Geometry: final body of the model. Coordinates: model frame, mm. Face numbers are marked on the shaded views. Coordinates: 2 decimals unless noted, no trailing zeros. Write each loop counter-clockwise with the first axis right and the second up, starting at its lowest first coordinate (ties: lowest second). Pieces come first, ordered by that corner, then holes. Notation, with made-up numbers: (-27.75, 82) -> (16.25, 82) arc R18 cw to (16.25, 89) -> close; hole circle Ø11 at (80, -23). An arc over 180 degrees is marked (long way). One line per item, written item: value.
```python
from build123d import *

# Parameters (mm, degrees)
F0_W      = 76.2
F0_H      = 146.05
F1_DEPTH  = 12.7
F2_R      = 5.08
F3_R      = 5.08
F4_DEPTH  = 2.54
F5_W      = 2.4973305091
F5_H      = 11.7452070117
F5_W_2    = 2.54
F5_W_3    = 2.9405460703
F6_DEPTH  = 2.54
F7_W      = 2.8808997013
F7_H      = 5.0969719887
F8_DEPTH  = 2.032
F9_W      = 1.4404498506
F9_H      = 5.0969719887
F10_DEPTH = 3.048
F11_W     = 2.54
F11_H     = 11.43
F12_DEPTH = 1.016
F13_W     = 2.54
F13_H     = 11.43
F14_DEPTH = 1.016
F16_DEPTH = 0.508
F17_W     = 15.7348513603
F17_H     = 10.4662538506
F17_H_2   = 4.2268524888
F18_DEPTH = 2.286
F19_W     = 18.1282758713
F19_H     = 1.7902922965
F19_H_2   = 2.54
F19_H_3   = 2.6172961119
F20_DEPTH = 2.286
F21_R     = 2.1027824112
F22_DEPTH = 2.286
F24_DEPTH = 1.27
F25_W     = 13.5468328476
F25_H     = 1.6100406647
F4_FACE_W = 66.04
F4_FACE_H = 135.89
F4_FACE_R = 6.0325
F26_DEPTH = 0.508
F27_R     = 1.3953400064
F28_DEPTH = 0.508
F30_DEPTH = 0.508
F31_W     = 6.604
F31_H     = 3.0624943002
F31_H_2   = 5.8275056998
F31_H_3   = 2.54
F32_DEPTH = 2.286
F34_DEPTH = 1.27
F35_W     = 24.4420864832
F35_H     = 11.2134301376
F36_DEPTH = 2.286
F39_R     = 2.3136513578
F40_DEPTH = 0.254
F42_DEPTH = 1.016
F43_DEPTH = 1.778
F44_W     = 2.54
F44_H     = 8.934661746
F45_DEPTH = 1.016


# Not quite as in the source:
# - the program builds the solid bodies; features that only make, move or delete a surface that nothing else refers to are left out


with BuildPart() as f1:
    # F0 (on Front) → F1 (new body)
    with BuildSketch(Plane.XZ):
        with Locations((38.1, 73.025)):
            Rectangle(F0_W, F0_H)
    extrude(amount=F1_DEPTH)

    # F2
    f2_edges = [f1.edges().sort_by_distance(p)[0] for p in [
        (0, -12.7, 73.025),
        (38.1, -12.7, 0),
        (76.2, -12.7, 73.025),
        (38.1, -12.7, 146.05),
    ]]
    fillet(f2_edges, radius=F2_R)

    # F3
    f3_edges = [f1.edges().sort_by_distance(p)[0] for p in [
        (0, 0, 73.025),
        (38.1, 0, 0),
        (76.2, 0, 73.025),
        (38.1, 0, 146.05),
    ]]
    fillet(f3_edges, radius=F3_R)

    # F4 (cut): a face of the model
    f4_faces = [f1.faces().sort_by_distance(p)[0] for p in [
        (38.1, -12.7, 73.025),
    ]]
    extrude(f4_faces, amount=-F4_DEPTH, mode=Mode.SUBTRACT)

    # F5 (on face) → F6 (cut)
    with BuildSketch(Plane(origin=(0, 0, 0), x_dir=(0, -1, 0), z_dir=(-1, 0, 0))):
        with Locations((3.8313347455, 127.8729029)):
            Rectangle(F5_W, F5_H)
        with Locations((6.35, 127.8729029)):
            Rectangle(F5_W_2, F5_H)
        with Locations((9.0902730352, 127.8729029)):
            Rectangle(F5_W_3, F5_H)
    extrude(amount=-F6_DEPTH, mode=Mode.SUBTRACT)

    # F7 (on face) → F8 (join)
    with BuildSketch(Plane(origin=(2.54, 0, 0), x_dir=(0, -1, 0), z_dir=(-1, 0, 0))):
        with Locations((6.2391965184, 127.6512891054)):
            Rectangle(F7_W, F7_H)
    extrude(amount=F8_DEPTH)

    # F9 (on face) → F10 (cut)
    with BuildSketch(Plane(origin=(0.508, 0, 0), x_dir=(0, -1, 0), z_dir=(-1, 0, 0))):
        with Locations((6.9594214438, 127.6512891054)):
            Rectangle(F9_W, F9_H)
    extrude(amount=-F10_DEPTH, mode=Mode.SUBTRACT)

    # F11 (on face) → F12 (join)
    with BuildSketch(Plane(origin=(0, 0, 0), x_dir=(0, -1, 0), z_dir=(-1, 0, 0))):
        with Locations((6.35, 112.3141669893)):
            Rectangle(F11_W, F11_H)
    extrude(amount=F12_DEPTH)

    # F13 (on face) → F14 (join)
    with BuildSketch(Plane(origin=(0, 0, 0), x_dir=(0, -1, 0), z_dir=(-1, 0, 0))):
        with Locations((6.35, 97.9860373998)):
            Rectangle(F13_W, F13_H)
    extrude(amount=F14_DEPTH)

    # F15 (on face) → F16 (cut)
    with BuildSketch(Plane.XZ.offset(10.16)):
        with BuildLine():
            ThreePointArc((44.1325, 12.7), (33.8343783425, 16.9656216575), (38.1, 6.6675))
            ThreePointArc((38.1, 6.6675), (42.3656216575, 8.4343783425), (44.1325, 12.7))
        make_face()
    extrude(amount=-F16_DEPTH, mode=Mode.SUBTRACT)

    # F17 (on face) → F18 (cut)
    with BuildSketch(Plane(origin=(0, 0, 0), x_dir=(1, 0, 0), z_dir=(0, 0, -1))):
        with Locations((14.6331973374, 6.6137255635)):
            Rectangle(F17_W, F17_H)
        with Locations((14.6331973374, 9.7334262444)):
            Rectangle(F17_W, F17_H_2)
    extrude(amount=-F18_DEPTH, mode=Mode.SUBTRACT)

    # F19 (on face) → F20 (cut)
    with BuildSketch(Plane(origin=(0, 0, 0), x_dir=(1, 0, 0), z_dir=(0, 0, -1))):
        with Locations((61.1127465963, 4.1848538518)):
            Rectangle(F19_W, F19_H)
        with Locations((61.1127465963, 6.35)):
            Rectangle(F19_W, F19_H_2)
        with Locations((61.1127465963, 8.9286480559)):
            Rectangle(F19_W, F19_H_3)
    extrude(amount=-F20_DEPTH, mode=Mode.SUBTRACT)

    # F21 (on face) → F22 (cut)
    with BuildSketch(Plane(origin=(0, 0, 2.286), x_dir=(1, 0, 0), z_dir=(0, 0, -1))):
        with Locations((14.4449183717, 6.7520015873)):
            Circle(F21_R)
    extrude(amount=-F22_DEPTH, mode=Mode.SUBTRACT)

    # F23 (on face) → F24 (cut)
    with BuildSketch(Plane(origin=(0, 0, 2.286), x_dir=(1, 0, 0), z_dir=(0, 0, -1))):
        with BuildLine():
            ThreePointArc((54.0211938972, 6.1539337039), (53.2591938972, 6.9159337039), (52.4971938972, 6.1539337039))
            Line((52.4971938972, 6.1539337039), (54.0211938972, 6.1539337039))
        make_face()
        with BuildLine():
            ThreePointArc((69.8944770451, 6.1539337039), (69.1324770451, 6.9159337039), (68.3704770451, 6.1539337039))
            Line((68.3704770451, 6.1539337039), (69.8944770451, 6.1539337039))
        make_face()
        with BuildLine():
            Line((69.8944770451, 6.1539337039), (68.3704770451, 6.1539337039))
            ThreePointArc((68.3704770451, 6.1539337039), (69.1324770451, 5.3919337039), (69.8944770451, 6.1539337039))
        make_face()
        with BuildLine():
            ThreePointArc((67.8202428575, 6.1539337039), (67.0582428575, 6.9159337039), (66.2962428575, 6.1539337039))
            Line((66.2962428575, 6.1539337039), (67.8202428575, 6.1539337039))
        make_face()
        with BuildLine():
            Line((67.8202428575, 6.1539337039), (66.2962428575, 6.1539337039))
            ThreePointArc((66.2962428575, 6.1539337039), (67.0582428575, 5.3919337039), (67.8202428575, 6.1539337039))
        make_face()
        with BuildLine():
            ThreePointArc((65.8047863002, 6.1539337039), (65.0427863002, 6.9159337039), (64.2807863002, 6.1539337039))
            Line((64.2807863002, 6.1539337039), (65.8047863002, 6.1539337039))
        make_face()
        with BuildLine():
            Line((65.8047863002, 6.1539337039), (64.2807863002, 6.1539337039))
            ThreePointArc((64.2807863002, 6.1539337039), (65.0427863002, 5.3919337039), (65.8047863002, 6.1539337039))
        make_face()
        with BuildLine():
            ThreePointArc((63.588320529, 6.1539337039), (62.826320529, 6.9159337039), (62.064320529, 6.1539337039))
            Line((62.064320529, 6.1539337039), (63.588320529, 6.1539337039))
        make_face()
        with BuildLine():
            Line((63.588320529, 6.1539337039), (62.064320529, 6.1539337039))
            ThreePointArc((62.064320529, 6.1539337039), (62.826320529, 5.3919337039), (63.588320529, 6.1539337039))
        make_face()
        with BuildLine():
            ThreePointArc((61.1659095342, 6.1539337039), (60.4039095342, 6.9159337039), (59.6419095342, 6.1539337039))
            Line((59.6419095342, 6.1539337039), (61.1659095342, 6.1539337039))
        make_face()
        with BuildLine():
            Line((61.1659095342, 6.1539337039), (59.6419095342, 6.1539337039))
            ThreePointArc((59.6419095342, 6.1539337039), (60.4039095342, 5.3919337039), (61.1659095342, 6.1539337039))
        make_face()
        with BuildLine():
            ThreePointArc((58.6699277813, 6.1539337039), (57.9079277813, 6.9159337039), (57.1459277813, 6.1539337039))
            Line((57.1459277813, 6.1539337039), (58.6699277813, 6.1539337039))
        make_face()
        with BuildLine():
            Line((58.6699277813, 6.1539337039), (57.1459277813, 6.1539337039))
            ThreePointArc((57.1459277813, 6.1539337039), (57.9079277813, 5.3919337039), (58.6699277813, 6.1539337039))
        make_face()
        with BuildLine():
            ThreePointArc((56.3848160858, 6.1539337039), (55.6228160858, 6.9159337039), (54.8608160858, 6.1539337039))
            Line((54.8608160858, 6.1539337039), (56.3848160858, 6.1539337039))
        make_face()
        with BuildLine():
            Line((56.3848160858, 6.1539337039), (54.8608160858, 6.1539337039))
            ThreePointArc((54.8608160858, 6.1539337039), (55.6228160858, 5.3919337039), (56.3848160858, 6.1539337039))
        make_face()
        with BuildLine():
            Line((54.0211938972, 6.1539337039), (52.4971938972, 6.1539337039))
            ThreePointArc((52.4971938972, 6.1539337039), (53.2591938972, 5.3919337039), (54.0211938972, 6.1539337039))
        make_face()
    extrude(amount=-F24_DEPTH, mode=Mode.SUBTRACT)

    # F25 (on face) + F4_face (on face) → F26 (cut)
    with BuildSketch(Plane.XZ.offset(9.652)):
        with Locations((38.1, 135.0751519203)):
            Rectangle(F25_W, F25_H)
    with BuildSketch(Plane(origin=(38.1, -10.16, 73.025), x_dir=(1, 0, 0), z_dir=(0, -1, 0))):
        Rectangle(F4_FACE_W, F4_FACE_H)
        with Locations((0, -60.325)):
            Circle(F4_FACE_R, mode=Mode.SUBTRACT)
    extrude(amount=-F26_DEPTH, mode=Mode.SUBTRACT)

    # F27 (on face) → F28 (cut)
    with BuildSketch(Plane.XZ.offset(9.652)):
        with Locations((25.323253125, 135.4901641607)):
            Circle(F27_R)
    extrude(amount=-F28_DEPTH, mode=Mode.SUBTRACT)

    # F29 (on face) → F30 (cut)
    with BuildSketch(Plane.XZ.offset(9.652)):
        with BuildLine():
            ThreePointArc((44.1325, 12.7), (33.8343783425, 16.9656216575), (38.1, 6.6675))
            ThreePointArc((38.1, 6.6675), (42.3656216575, 8.4343783425), (44.1325, 12.7))
        make_face()
    extrude(amount=-F30_DEPTH, mode=Mode.SUBTRACT)

    # F31 (on face) → F32 (cut)
    with BuildSketch(Plane(origin=(0, 0, 0), x_dir=(1, 0, 0), z_dir=(0, 0, -1))):
        with Locations((34.9296401281, 3.5487528499)):
            Rectangle(F31_W, F31_H)
        with Locations((41.5336401281, 10.5337528499)):
            Rectangle(F31_W, F31_H_2)
        with Locations((41.5336401281, 3.5487528499)):
            Rectangle(F31_W, F31_H)
        with Locations((34.9296401281, 6.35)):
            Rectangle(F31_W, F31_H_3)
        with Locations((41.5336401281, 6.35)):
            Rectangle(F31_W, F31_H_3)
        with Locations((34.9296401281, 10.5337528499)):
            Rectangle(F31_W, F31_H_2)
    extrude(amount=-F32_DEPTH, mode=Mode.SUBTRACT)

    # F33 (on face) → F34 (cut)
    with BuildSketch(Plane(origin=(0, 0, 2.286), x_dir=(1, 0, 0), z_dir=(0, 0, -1))):
        Polygon((34.6526485043, 7.9915548147), (34.6526485043, 6.9400710721), (34.6526485043, 5.8885873295), (41.810631752, 5.8885873295), (41.810631752, 7.9915548147), align=None)
    extrude(amount=-F34_DEPTH, mode=Mode.SUBTRACT)

    # F35 (on face) → F36 (cut)
    with BuildSketch(Plane(origin=(0, 0, 0), x_dir=(-1, 0, 0), z_dir=(0, 1, 0))):
        with Locations((-58.8989567584, 135.3632849312)):
            Rectangle(F35_W, F35_H)
    extrude(amount=-F36_DEPTH, mode=Mode.SUBTRACT)

    # F39 (on face) → F40 (cut)
    with BuildSketch(Plane(origin=(0, -2.286, 0), x_dir=(-1, 0, 0), z_dir=(0, 1, 0))):
        with Locations((-53.6911524832, 134.4103217125)):
            Circle(F39_R)
    extrude(amount=-F40_DEPTH, mode=Mode.SUBTRACT)

    # F41 (on face) → F42 (cut)
    with BuildSketch(Plane(origin=(0, 0, 0), x_dir=(-1, 0, 0), z_dir=(0, 1, 0))):
        with BuildLine():
            ThreePointArc((-38.1, 122.8167432735), (-46.1358037085, 103.4165969759), (-26.7356574109, 111.4524006844))
            ThreePointArc((-26.7356574109, 111.4524006844), (-30.0641962915, 119.4882043929), (-38.1, 122.8167432735))
        make_face()
        with BuildLine():
            ThreePointArc((-26.7356574109, 111.4524006844), (-30.0641962915, 119.4882043929), (-38.1, 122.8167432735))
            ThreePointArc((-38.1, 122.8167432735), (-46.1358037085, 103.4165969759), (-26.7356574109, 111.4524006844))
        make_face()
    extrude(amount=-F42_DEPTH, mode=Mode.SUBTRACT)

    # F43 (cut): a face of the model
    f43_faces = [f1.faces().sort_by_distance(p)[0] for p in [
        (38.1, -1.016, 111.4524006844),
    ]]
    extrude(f43_faces, amount=-F43_DEPTH, mode=Mode.SUBTRACT)

    # F44 (on face) → F45 (join)
    with BuildSketch(Plane.YZ.offset(76.2)):
        with Locations((-6.35, 115.3773292899)):
            Rectangle(F44_W, F44_H)
    extrude(amount=F45_DEPTH)


solid = f1.part
```
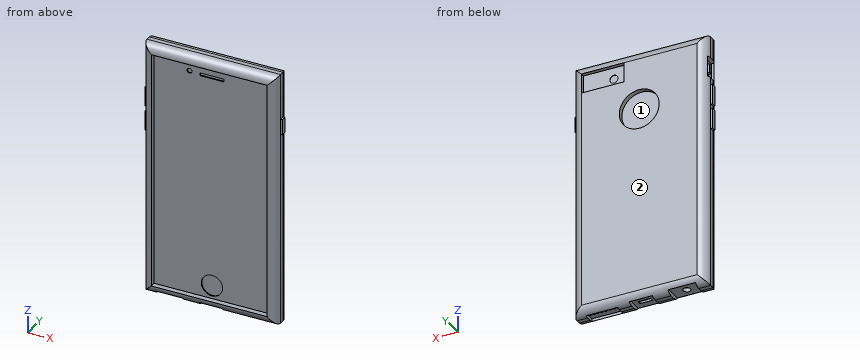
(1) Pull-direction query (Z, two-part tool) for the marked faces 1 and 2; classes: released by +Z, released by -Z, zero draft, split by the parting line, or undercut.
Responses:
face 1: undercut
face 2: zero draft
(2) Section C-C (z = 9.5). Return the cut outline in (x, y), then the cut area to 3 significant figures.
Responses:
outline: (0, -7.62) arc R5.08 ccw to (5.08, -12.7) -> (5.08, -9.65) -> (32.99, -9.65) -> (32.99, -9.14) -> (43.21, -9.14) -> (43.21, -9.65) -> (71.12, -9.65) -> (71.12, -12.7) arc R5.08 ccw to (76.2, -7.62) -> (76.2, -5.08) arc R5.08 ccw to (71.12, 0) -> (5.08, 0) arc R5.08 ccw to (0, -5.08) -> close
area: 739 mm2
(3) Section B-B (z = 69.5). Return the cut outline in (x, y), then the cut area to 3 significant figures.
Responses:
outline: (0, -7.62) arc R5.08 ccw to (5.08, -12.7) -> (5.08, -9.65) -> (71.12, -9.65) -> (71.12, -12.7) arc R5.08 ccw to (76.2, -7.62) -> (76.2, -5.08) arc R5.08 ccw to (71.12, 0) -> (5.08, 0) arc R5.08 ccw to (0, -5.08) -> close
area: 744 mm2
(4) Line query: line 1 (Y direction, x = 6.5, z = 55.5); line 2 (Y direction, x = 40.5, z = 122); line 3 (Z direction, x = 21, y = -10.75). Output: solid intervals per line, ascending. Write a range as [from, to].
Responses:
line 1: y = [-9.65, 0]
line 2: y = [-9.65, -2.79]
line 3: z = [2.29, 5.08], [140.97, 144.97]
(5) Section D-D (x = 40). Return the cut outline in (y, z).
Responses:
outline: (-12.7, 5.08) arc R5.08 ccw to (-11.86, 2.29) -> (-7.99, 2.29) -> (-7.99, 3.56) -> (-5.89, 3.56) -> (-5.89, 2.29) -> (-2.02, 2.29) -> (-2.02, 1.03) arc R5.08 ccw to (0, 5.08) -> (0, 100.25) -> (-2.79, 100.25) -> (-2.79, 122.66) -> (0, 122.66) -> (0, 140.97) arc R5.08 ccw to (-5.08, 146.05) -> (-7.62, 146.05) arc R5.08 ccw to (-12.7, 140.97) -> (-9.65, 140.97) -> (-9.65, 135.88) -> (-9.14, 135.88) -> (-9.14, 134.27) -> (-9.65, 134.27) -> (-9.65, 18.43) -> (-9.14, 18.43) -> (-9.14, 6.97) -> (-9.65, 6.97) -> (-9.65, 5.08) -> close
(6) First-contact query: pin 1 (0.9 mm diameter, centred on y = -10.5, z = 47, fed in from +X); pin 2 (0.5 mm diameter, centred on x = 3, z = 127.5, fed in from +Y); pin 3 (4 mm diameter, centred on y = -7, z = 36.5, fed in from +X). Flat tips, straight axial feed; report the tip coordinate or a pass-through.
Responses:
pin 1: stops at x = 75.58
pin 2: stops at y = -0.34
pin 3: stops at x = 76.2
